```python
from build123d import *

# Parameters (mm, degrees)
SKETCH_1_R      = 4
SKETCH_1_R_2    = 1.1
EXTRUDE_2_DEPTH = 6.6
SKETCH_2_W      = 6.666666666
SKETCH_2_H      = 2.2
EXTRUDE_3_DEPTH = 3


with BuildPart() as part:
    # 草图1 → 凸台-拉伸2 (new body)
    with BuildSketch(Plane(origin=(0, 0, 0), x_dir=(1, 0, 0), z_dir=(0, 1, 0))):
        with BuildLine():
            Line((-10, -17), (10, -17))
            Line((10, -17), (10, 0))
            ThreePointArc((10, 0), (8.100154011, 5.864086033), (3.122498999, 9.5))
            Line((3.122498999, 9.5), (-3.122498999, 9.5))
            ThreePointArc((-3.122498999, 9.5), (-8.100154011, 5.864086033), (-10, 0))
            Line((-10, 0), (-10, -17))
        make_face()
        with Locations(Location((0, 0, 0), (0, 0, 270))):
            Circle(SKETCH_1_R, mode=Mode.SUBTRACT)
        with Locations(Location((-7, 0, 0), (0, 0, 270))):
            Circle(SKETCH_1_R_2, mode=Mode.SUBTRACT)
        with Locations(Location((0, 7, 0), (0, 0, 270))):
            Circle(SKETCH_1_R_2, mode=Mode.SUBTRACT)
        with Locations(Location((7, 0, 0), (0, 0, 270))):
            Circle(SKETCH_1_R_2, mode=Mode.SUBTRACT)
        with Locations(Location((0, -7, 0), (0, 0, 270))):
            Circle(SKETCH_1_R_2, mode=Mode.SUBTRACT)
    extrude(amount=EXTRUDE_2_DEPTH)

    # 草图2 → 凸台-拉伸3 (add)
    with BuildSketch(Plane.XY.offset(17)):
        with Locations((0, 3.3)):
            Rectangle(SKETCH_2_W, SKETCH_2_H)
    extrude(amount=EXTRUDE_3_DEPTH)


solid = part.part
```
Input: part model. Units: mm. Frame: model coordinates. A direction names the side the tool comes from. Round coordinates to 2 decimals unless told otherwise and drop trailing zeros. Loops run counter-clockwise (first coordinate to the right, second up) from the corner with the lowest first, then second, coordinate; pieces in that order, holes last. Notation, with made-up numbers: (7, 68.5) - (48, 68.5) arc R20 cw to (48, 73.5) - close; hole circle Ø9 at (-27, 1.25). An arc over 180 degrees is marked (long way). One line per item, written item: value. Start each with the question number.
(1) Section D-D, the plane x = -7. Return loops of the section in (y, z).
(2) Draft query along Z for faces 1 (the cylindrical face through (8, 3, -6)), 2 (the cylindrical face through (-0.421, 3.254, 8.016)), 3 (the cylindrical face through (-0.421, 3.254, -5.984)), 4 (the flat face through (0, 4.4, 18)). Return one class per face: +Z half, -Z half, draft (parallel to the pull), parting line (faces both ways), or undercut.
(3) Access query for faces 5 (the flat face through (3.333, 3, 18)), 6 (the flat face through (0, 2.2, 18)), 7 (the flat face through (-3.333, 3, 18)). Directions: +Z, -Z, +X, -X, +Y, -Y. A direction counts if a zero-diameter tool reaches every point of the face in a straight line with its end or side. Return the directions, or none.
(4) Contact query for flat-ended pins moving along their axis: P1, Ø1.8, axis at y = 3, z = 18, coming from the -X side; P2, Ø0.9, axis at x = -1, z = 18.5, coming from the +Y side; P3, Ø0.7, axis at y = 3.5, z = 18.5, coming from the +X side. Output: stop coordinate, or through.
(5) Section C-C, the plane y = 3.75. Return loops of the section in (x, z), plus the area to 3 significant figures.
(6) Section A-A, the plane z = 7. Return loops of the section in (x, y).
(7) Ray query, line 1 (X direction, y = 3.75, z = 0); line 2 (Z direction, x = 2.5, y = 3.5); line 3 (X direction, y = 3, z = 7). Return the intervals inside material, ascending. Write a range as [from, to].
(8) Section B-B, the plane x = 0. Return loops of the section in (y, z), plus the area to 3 significant figures.
Results below:
1. outline: (0, -7.14) - (6.6, -7.14) - (6.6, -1.1) - (0, -1.1) - close; (0, 1.1) - (6.6, 1.1) - (6.6, 17) - (0, 17) - close
2. face 1: -Z half
2. face 2: undercut
2. face 3: undercut
2. face 4: draft
3. face 5: +Z, +X, +Y, -Y
3. face 6: +Z, +X, -X, -Y
3. face 7: +Z, -X, +Y, -Y
4. P1: x = -3.33
4. P2: y = 4.4
4. P3: x = 3.33
5. outline: (-10, 0) arc R10 ccw to (-3.12, -9.5) - (3.12, -9.5) arc R10 ccw to (10, 0) - (10, 17) - (3.33, 17) - (3.33, 20) - (-3.33, 20) - (-3.33, 17) - (-10, 17) - close; hole circle Ø2.2 at (-7, 0); hole circle Ø8 at (0, 0); hole circle Ø2.2 at (0, -7); hole circle Ø2.2 at (0, 7); hole circle Ø2.2 at (7, 0)
5. area: 450 mm^2
6. outline: (-10, 0) - (-1.1, 0) - (-1.1, 6.6) - (-10, 6.6) - close; (1.1, 0) - (10, 0) - (10, 6.6) - (1.1, 6.6) - close
7. line 1: [-10, -8.1], [-5.9, -4], [4, 5.9], [8.1, 10]
7. line 2: [-9.5, -3.12], [3.12, 20]
7. line 3: [-10, -1.1], [1.1, 10]
8. outline: (0, -9.5) - (6.6, -9.5) - (6.6, -8.1) - (0, -8.1) - close; (0, -5.9) - (6.6, -5.9) - (6.6, -4) - (0, -4) - close; (0, 4) - (6.6, 4) - (6.6, 5.9) - (0, 5.9) - close; (0, 8.1) - (6.6, 8.1) - (6.6, 17) - (4.4, 17) - (4.4, 20) - (2.2, 20) - (2.2, 17) - (0, 17) - close
8. area: 99.7 mm^2
